Source: CAD feature listing. Evaluate the final solid. Frame: model axes, mm. Face numbers are marked on the shaded views. A direction names the side the tool comes from. Give positions to 0.01 mm unless a question says otherwise; leave off trailing zeros. Loops run counter-clockwise (first coordinate to the right, second up) from the corner with the lowest first, then second, coordinate; pieces in that order, holes last. Notation, with made-up numbers: M 57,78.25 L 104,78.25 A30 cw 104,116.25 Z; hole C 68,-12 d10. An arc over 180 degrees is marked long. Answer in a Markdown table with one row per item.
```python
from build123d import *

# Parameters (mm, degrees)
PAD_DEPTH       = 9
SKETCH001_W     = 26.1
SKETCH001_H     = 34.4
POCKET_DEPTH    = 3
SKETCH002_R     = 22.22
PAD001_DEPTH    = 3
SKETCH003_R     = 24.44
PAD002_DEPTH    = 3
SKETCH004_R     = 26.6
PAD003_DEPTH    = 3
SKETCH005_R     = 28
PAD004_DEPTH    = 3
SKETCH006_R     = 29
PAD005_DEPTH    = 3
SKETCH007_R     = 29
PAD006_DEPTH    = 3
SKETCH008_R     = 29
PAD007_DEPTH    = 3
SKETCH009_W     = 17
SKETCH009_H     = 24
POCKET001_DEPTH = 3
SKETCH010_W     = 16
SKETCH010_H     = 9
POCKET002_DEPTH = 7
SKETCH011_W     = 20
SKETCH011_H     = 10
POCKET003_DEPTH = 3


with BuildPart() as part:
    # Sketch → Pad (new body)
    with BuildSketch(Plane.XY):
        Polygon((44, 0), (22, 38.105118), (-22, 38.105118), (-44, 0), (-22, -38.105118), (22, -38.105118), align=None)
    extrude(amount=PAD_DEPTH)

    # Sketch001 (on Face8 of Pad) → Pocket (cut)
    with BuildSketch(Plane.XY.offset(9)):
        with Locations((0, -13.905118)):
            Rectangle(SKETCH001_W, SKETCH001_H)
    extrude(amount=-POCKET_DEPTH, mode=Mode.SUBTRACT)

    # Sketch002 (on Face5 of Pocket) → Pad001 (join)
    with BuildSketch(Plane.XY.offset(9)):
        Polygon((22, 38.105118), (-22, 38.105118), (-44, 0), (-22, -38.105118), (22, -38.105118), (44, 0), align=None)
        Circle(SKETCH002_R, mode=Mode.SUBTRACT)
    extrude(amount=PAD001_DEPTH)

    # Sketch003 (on Face14 of Pad001) → Pad002 (join)
    with BuildSketch(Plane.XY.offset(12)):
        Polygon((40, 0), (20, 34.641016), (-20, 34.641016), (-40, 0), (-20, -34.641016), (20, -34.641016), align=None)
        Circle(SKETCH003_R, mode=Mode.SUBTRACT)
    extrude(amount=PAD002_DEPTH)

    # Sketch004 (on Face21 of Pad002) → Pad003 (join)
    with BuildSketch(Plane.XY.offset(15)):
        Polygon((41, 0), (20.5, 35.507042), (-20.5, 35.507042), (-41, 0), (-20.5, -35.507042), (20.5, -35.507042), align=None)
        Circle(SKETCH004_R, mode=Mode.SUBTRACT)
    extrude(amount=PAD003_DEPTH)

    # Sketch005 (on Face28 of Pad003) → Pad004 (join)
    with BuildSketch(Plane.XY.offset(18)):
        Polygon((19, 32.908965), (-19, 32.908965), (-38, 0), (-19, -32.908965), (19, -32.908965), (38, 0), align=None)
        Circle(SKETCH005_R, mode=Mode.SUBTRACT)
    extrude(amount=PAD004_DEPTH)

    # Sketch006 (on Face35 of Pad004) → Pad005 (join)
    with BuildSketch(Plane.XY.offset(21)):
        Polygon((39, 0), (19.5, 33.774991), (-19.5, 33.774991), (-39, 0), (-19.5, -33.774991), (19.5, -33.774991), align=None)
        Circle(SKETCH006_R, mode=Mode.SUBTRACT)
    extrude(amount=PAD005_DEPTH)

    # Sketch007 (on Face42 of Pad005) → Pad006 (join)
    with BuildSketch(Plane.XY.offset(24)):
        Polygon((36, 0), (18, 31.176915), (-18, 31.176915), (-36, 0), (-18, -31.176915), (18, -31.176915), align=None)
        Circle(SKETCH007_R, mode=Mode.SUBTRACT)
    extrude(amount=PAD006_DEPTH)

    # Sketch008 (on Face49 of Pad006) → Pad007 (join)
    with BuildSketch(Plane.XY.offset(27)):
        Polygon((37, 0), (18.5, 32.04294), (-18.5, 32.04294), (-37, 0), (-18.5, -32.04294), (18.5, -32.04294), align=None)
        Circle(SKETCH008_R, mode=Mode.SUBTRACT)
    extrude(amount=PAD007_DEPTH)

    # Sketch009 (on Face74 of Pad007) → Pocket001 (cut)
    with BuildSketch(Plane.XY.offset(6)):
        with Locations((0, -8.705118)):
            Rectangle(SKETCH009_W, SKETCH009_H)
    extrude(amount=-POCKET001_DEPTH, mode=Mode.SUBTRACT)

    # Sketch010 (on Face12 of Pocket001) → Pocket002 (cut)
    with BuildSketch(Plane.XZ.offset(38.105118)):
        with Locations((0, 7.5)):
            Rectangle(SKETCH010_W, SKETCH010_H)
    extrude(amount=-POCKET002_DEPTH, mode=Mode.SUBTRACT)

    # Sketch011 (on Face40 of Pocket002) → Pocket003 (cut)
    with BuildSketch(Plane.XY.offset(9)):
        with Locations((0, 17.22)):
            Rectangle(SKETCH011_W, SKETCH011_H)
    extrude(amount=-POCKET003_DEPTH, mode=Mode.SUBTRACT)


solid = part.part
```
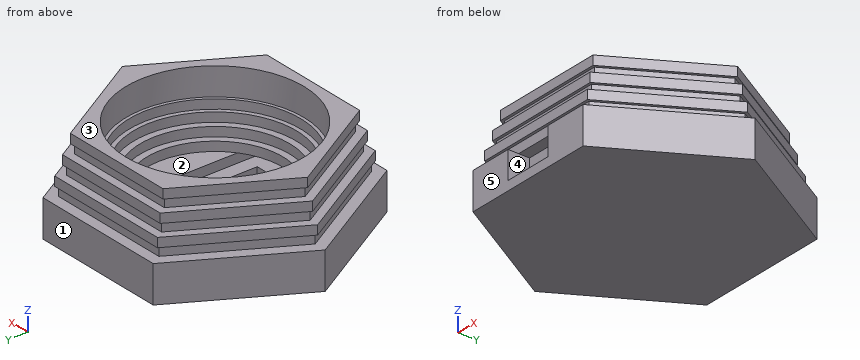
1) Section C-C, the plane x = -31.5. Return loops of the section in (y, z).
Reply:
| item | result |
|---|---|
| outline | M -21.65,0 L 21.65,0 L 21.65,12 L 14.72,12 L 14.72,15 L 16.45,15 L 16.45,18 L 11.26,18 L 11.26,21 L 12.99,21 L 12.99,24 L 7.79,24 L 7.79,27 L 9.53,27 L 9.53,30 L -9.53,30 L -9.53,27 L -7.79,27 L -7.79,24 L -12.99,24 L -12.99,21 L -11.26,21 L -11.26,18 L -16.45,18 L -16.45,15 L -14.72,15 L -14.72,12 L -21.65,12 Z |
2) Section A-A, the plane z = 25. Return loops of the section in (x, y), then the cut area to 3 significant figures.
Reply:
| item | result |
|---|---|
| outline | M -36,0 L -18,-31.18 L 18,-31.18 L 36,0 L 18,31.18 L -18,31.18 Z; hole C 0,0 d58 |
| area | 725 mm² |
3) Set-up query: the marked faces 1 and 2. Return all of +Z, -Z, +X, -X, +Y, -Y with unobstructed straight access to the full face (end or side cutting, diameter ignored); none if empty.
Reply:
| item | result |
|---|---|
| face 1 | +Z, -Z, +X, -X, +Y |
| face 2 | +Z |
4) Material intervals for L1, parallel to Y at x = -4, z = 6.5; L2, parallel to X at y = 0, z = 10.6; L3, parallel to Y at x = 0, z = 16.3, sorted ascending.
Reply:
| item | result |
|---|---|
| L1 | y = 3.29 to 12.22, 22.22 to 38.11 |
| L2 | x = -44 to -22.22, 22.22 to 44 |
| L3 | y = -35.51 to -26.6, 26.6 to 35.51 |
5) Section B-B, the plane z = 17. Return loops of the section in (x, y), then the cut area to 3 significant figures.
Reply:
| item | result |
|---|---|
| outline | M -41,0 L -20.5,-35.51 L 20.5,-35.51 L 41,0 L 20.5,35.51 L -20.5,35.51 Z; hole C 0,0 d53.2 |
| area | 2,140 mm² |
6) Pull-direction query (Z, two-part tool) for the marked faces 3, 4 and 5; classes: released by +Z, released by -Z, zero draft, split by the parting line, or undercut.
Reply:
| item | result |
|---|---|
| face 3 | released by +Z |
| face 4 | undercut |
| face 5 | zero draft |
7) Pin query (flat end, axial travel): pin 1 Ø4 at (y, z) = (26, 14.5) entering from -X; pin 2 Ø1.9 at (x, y) = (5, 21) entering from -Z; pin 3 Ø0.9 at (y, z) = (-7.5, 7) entering from -X; pin 4 Ø0.9 at (x, z) = (9, 16.5) entering from -Y. Return the tip coordinate at first contact, or that it passes through.
Reply:
| item | result |
|---|---|
| pin 1 | stops at x = -27.11 |
| pin 2 | stops at z = 0 |
| pin 3 | stops at x = -39.93 |
| pin 4 | stops at y = -35.51 |
